Autodesk Inventor part; units mm, degrees
ref_plane "YZ Plane" through (0, 0, 0) normal (1, 0, 0) x (0, 1, 0)
ref_plane "XZ Plane" through (0, 0, 0) normal (0, 1, 0) x (-1, 0, 0)
ref_plane "XY Plane" through (0, 0, 0) normal (0, 0, 1) x (1, 0, 0)
sketch "Sketch1" plane through (0, 0, 0) normal (0, 1, 0) x (-1, 0, 0)
  line L0 (0, 0) -> (71.374, 0)
  line L1 (71.374, 0) -> (71.374, -19.05)
  line L2 (0, -19.05) -> (0, 0)
  line L3 (71.374, -19.05) -> (71.374, -31.75)
  line L4 (71.374, -31.75) -> (0, -31.75)
  line L5 (0, -31.75) -> (0, -19.05)
  line L6 (71.374, 0) -> (71.374, -6.35)
  line L7 (71.374, -6.35) -> (87.352, -6.35)
  line L8 (71.374, -31.75) -> (71.374, -25.4)
  line L9 (71.374, -25.4) -> (87.352, -25.4)
  line L10 (71.374, -6.35) -> (-10.213, -6.35)
  line L11 (71.374, -25.4) -> (-10.213, -25.4)
  dimension "d0" = 71.374
  dimension "d1" = 19.05
  dimension "d2" = 12.7
  dimension "d3" = 6.35
  dimension "d4" = 6.35
extrude "Extrusion1" add sketch "Sketch1" along normal blind 3.048
sketch "Sketch2" plane through (0, 3.048, 0) normal (0, 1, 0) x (1, 0, 0)
  line L0 (-71.374, 0) -> (0, 0)
  line L1 (0, 0) -> (0, 6.35)
  line L2 (0, 0) -> (0, 31.75)
  line L3 (0, 6.35) -> (-71.374, 6.35)
  line L4 (-71.374, 31.75) -> (-71.374, 0)
  line L5 (-71.374, 31.75) -> (-71.374, 25.4)
  line L6 (-71.374, 25.4) -> (0, 25.4)
  line L7 (0, 6.35) -> (0, 10.7315)
  line L8 (0, 10.7315) -> (-19.0957, 10.7315)
  line L9 (0, 25.4) -> (0, 21.0185)
  line L10 (0, 21.0185) -> (-20.1254, 21.0185)
  line L11 (0, 10.7315) -> (-22.7876, 10.7315)
  line L12 (-71.374, 6.35) -> (-71.374, 10.7315)
  line L13 (-71.374, 10.7315) -> (-48.5864, 10.7315)
  line L14 (-48.5864, 10.7315) -> (-48.5864, 21.0185)
  line L15 (-48.5864, 21.0185) -> (-71.374, 21.0185)
  line L16 (-22.7876, 10.7315) -> (-22.7876, 21.0185)
  line L17 (-22.7876, 21.0185) -> (-20.1254, 21.0185)
  line L18 (-22.7876, 10.7315) -> (-48.5864, 10.7315)
  line L19 (-48.5864, 21.0185) -> (-22.7876, 21.0185)
  line L20 (-21.5176, 10.7315) -> (-21.5176, 21.0185)
  line L21 (-49.8564, 10.7315) -> (-49.8564, 21.0185)
  line L22 (-22.7876, 9.4615) -> (-48.5864, 9.4615)
  line L23 (-48.5864, 22.2885) -> (-22.7876, 22.2885)
  line L24 (-48.5864, 9.4615) -> (-49.8564, 9.4615)
  line L25 (-49.8564, 9.4615) -> (-49.8564, 10.7315)
  line L26 (-49.8564, 21.0185) -> (-49.8564, 22.2885)
  line L27 (-49.8564, 22.2885) -> (-48.5864, 22.2885)
  line L28 (-22.7876, 22.2885) -> (-21.5176, 22.2885)
  line L29 (-21.5176, 22.2885) -> (-21.5176, 21.0185)
  line L30 (-21.5176, 10.7315) -> (-21.5176, 9.4615)
  line L31 (-22.7876, 9.4615) -> (-21.5176, 9.4615)
  dimension "d7" = 6.35
  dimension "d8" = 6.35
  dimension "d9" = 4.3815
  dimension "d10" = 4.3815
  dimension "d11" = 22.7876
  dimension "d12" = 4.3815
  dimension "d13" = 22.7876
  dimension "d14" = 1.27
  dimension "d15" = 1.27
  dimension "d16" = 1.27
  dimension "d17" = 1.27
extrude "Extrusion2" cut sketch "Sketch2" against normal blind 19.177 contours L21 L15 L14 L13 | L13 L18 L11 L30 L31 L22 L24 L25 | L26 L27 L23 L28 L29 L17 L19 L15 | L14 L19 L16 L18 | L11 L16 L17 L20
sketch "Sketch3" plane through (0, 0, 0) normal (0, -1, 0) x (1, 0, 0)
  line L0 (0, -31.75) -> (-71.374, -31.75)
  line L1 (0, -31.75) -> (-3.048, -31.75)
  line L2 (-3.048, -31.75) -> (-3.048, 0)
  line L3 (-3.048, 0) -> (0, 0)
  line L4 (0, 0) -> (0, -31.75)
  line L5 (0, 0) -> (0, -31.75)
  line L6 (-71.374, -31.75) -> (-68.1711, -31.75)
  line L7 (-68.1711, -31.75) -> (-68.1711, 0)
  line L8 (-71.374, 0) -> (0, 0)
  line L9 (-71.374, 0) -> (-68.1711, 0)
  line L10 (-71.374, 0) -> (-71.374, -31.75)
  dimension "d20" = 3.048
extrude "Extrusion3" add sketch "Sketch3" along normal blind 12.7 contours L0 L2 L3 L4 | L0 L10 L8 L7
sketch "Sketch4" plane through (0, 3.048, 0) normal (1, 0, 0) x (0, 0, -1)
  line L0 (0, -15.748) -> (0, 0)
  line L1 (0, 0) -> (0, -15.748)
  line L2 (0, -15.748) -> (0, -3.048)
  line L3 (0, -3.048) -> (31.75, -3.048)
  line L4 (0, -3.048) -> (31.75, -3.048)
  line L5 (31.75, -3.048) -> (31.75, -15.748)
  line L6 (31.75, -15.748) -> (0, -15.748)
  line L7 (0, -15.748) -> (0, -10.7569)
  line L8 (0, -10.7569) -> (31.75, -10.7569)
  line L9 (0, -3.048) -> (0, -8.0429)
  line L10 (0, -8.0429) -> (31.75, -8.0429)
  line L11 (0, -10.7569) -> (0, -9.398)
  line L12 (0, -9.398) -> (6.35, -9.398)
  circle A0 centre (6.35, -9.398) radius 1.3551
  line L13 (31.75, -9.398) -> (25.4, -9.398)
  circle A1 centre (25.4, -9.398) radius 1.3551
  dimension "d23" = 12.7
  dimension "d24" = 4.9911
  dimension "d25" = 4.9949
  dimension "d26" = 31.75
  dimension "d27" = 1.3589
  dimension "d28" = 6.35
  dimension "d29" = 6.35
extrude "Extrusion4" cut sketch "Sketch4" against normal blind 96.8375 contours A0 | A1
properties part number "Power Switch Mount"
Input: part model. Units: mm. Frame: model coordinates. A direction names the side the tool comes from. Coordinates: 2 decimals unless noted, no trailing zeros. Write each loop counter-clockwise with the first axis right and the second up, starting at its lowest first coordinate (ties: lowest second). Pieces come first, ordered by that corner, then holes. Notation, with made-up numbers: M 78.5,43.25 L 127.5,43.25 A14 ccw 127.5,66.25 Z; hole C 29.25,89 d11. An arc over 180 degrees is marked long. Answer as a JSON object with one key per item and string values. Group by question number.
(1) Set-up query: faces 1 (the face through (-2, -12.7, -16)), 2 (the face through (-35, 2, -9.462)), 3 (the face through (-68.171, -6, -16)). Return all of +Z, -Z, +X, -X, +Y, -Y with unobstructed straight access to the full face (end or side cutting, diameter ignored); none if empty.
(2) Section C-C on z = -6.5. Output: boundary loops of the cut face in (x, y).
(3) Contact query for flat-ended pins moving along their axis: P1, Ø8, axis at y = -1, z = -20, coming from the +X side; P2, Ø10, axis at x = -54, z = -7, coming from the -Y side; P3, Ø6, axis at x = -7.5, y = -9, coming from the -Z side. Output: stop coordinate, or through.
(4) Ray query, line 1 along Z through (x, y) = (-0.7, -6.35); line 2 along Y through (x, z) = (-0.6, -6.35); line 3 along X through (y, z) = (-8.75, -23). Return the intervals inside material, ascending. Write a range as [from, to].
(5) Section D-D on z = -29. Output: boundary loops of the cut face in (x, y).
(6) Section A-A on y = -6.35. Output: boundary loops of the cut face in (x, z).
(7) Mould query, pull axis Y, two halves, no side actions, for faces 4 (the face through (-1.5, -5.21, -7.08)), 5 (the face through (-3.048, -6, -16)), 6 (the face through (-35, 3.048, -23)), 7 (the face through (-69.75, -5.21, -7.08)). Classes: pulls with the +Y half, pulls with the -Y half, needs draft (parallel to the pull), parting line crosses it, or undercut.
(8) Section B-B on z = -10.5. Output: boundary loops of the cut face in (x, y), plus the area to 3 significant figures.
Result set:
{
 "1": {"face 1": "+Z, -Z, +X, -X, -Y", "face 2": "+Y, -Y", "face 3": "+Z, -Z, -Y"},
 "2": {"outline": "M -71.37,-12.7 L -68.17,-12.7 L -68.17,-7.7 L -71.37,-7.7 Z; M -71.37,-5 L -68.17,-5 L -68.17,0 L -3.05,0 L -3.05,-5 L 0,-5 L 0,3.05 L -71.37,3.05 Z; M -3.05,-12.7 L 0,-12.7 L 0,-7.7 L -3.05,-7.7 Z"},
 "3": {"P1": "stops at x = 0", "P2": "stops at y = 0", "P3": "passes through"},
 "4": {"line 1": "z = [-31.75, -26.76], [-24.04, -7.71], [-4.99, 0]", "line 2": "y = [-12.7, -7.71], [-4.99, 3.05]", "line 3": "x = [-71.37, -68.17], [-3.05, 0]"},
 "5": {"outline": "M -71.37,-12.7 L -68.17,-12.7 L -68.17,0 L -3.05,0 L -3.05,-12.7 L 0,-12.7 L 0,3.05 L -71.37,3.05 Z"},
 "6": {"outline": "M -71.37,-31.75 L -68.17,-31.75 L -68.17,-26.76 L -71.37,-26.76 Z; M -71.37,-24.04 L -68.17,-24.04 L -68.17,-7.71 L -71.37,-7.71 Z; M -71.37,-4.99 L -68.17,-4.99 L -68.17,0 L -71.37,0 Z; M -3.05,-31.75 L 0,-31.75 L 0,-26.76 L -3.05,-26.76 Z; M -3.05,-24.04 L 0,-24.04 L 0,-7.71 L -3.05,-7.71 Z; M -3.05,-4.99 L 0,-4.99 L 0,0 L -3.05,0 Z"},
 "7": {"face 4": "undercut", "face 5": "needs draft", "face 6": "pulls with the +Y half", "face 7": "undercut"},
 "8": {"outline": "M -71.37,-12.7 L -68.17,-12.7 L -68.17,0 L -49.86,0 L -49.86,3.05 L -71.37,3.05 Z; M -21.52,0 L -3.05,0 L -3.05,-12.7 L 0,-12.7 L 0,3.05 L -21.52,3.05 Z", "area": "211 mm2"}
}
